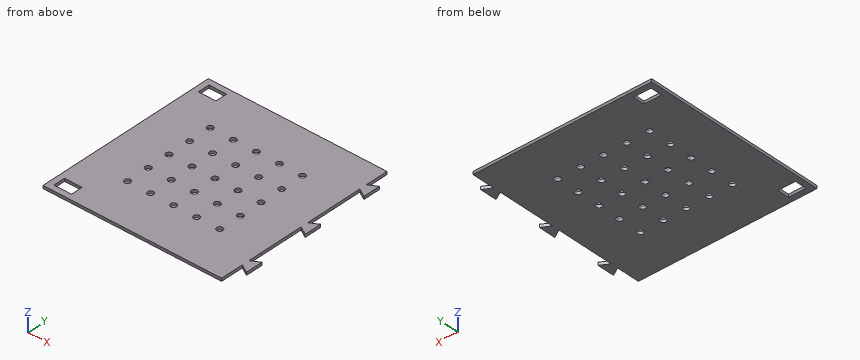
from build123d import *

# Parameters (mm, degrees)
SKETCH_W        = 155
SKETCH_H        = 160
PAD_DEPTH       = 2.5
SKETCH001_W     = 15.25
SKETCH001_H     = 10.25
POCKET_DEPTH    = 2.5
SKETCH002_R     = 2.625
POCKET001_DEPTH = 2.5
PAD001_DEPTH    = 2.5


with BuildPart() as part:
    # Sketch → Pad (new body)
    with BuildSketch(Plane.XY):
        with Locations((0.10674, -30.909095)):
            Rectangle(SKETCH_W, SKETCH_H)
    extrude(amount=PAD_DEPTH)

    # Sketch001 (on Face6 of Pad) → Pocket (cut)
    with BuildSketch(Plane.XY.offset(2.5)):
        with Locations((-64.76826, 38.965905)):
            Rectangle(SKETCH001_W, SKETCH001_H)
        with Locations((-64.76826, -100.784095)):
            Rectangle(SKETCH001_W, SKETCH001_H)
    extrude(amount=-POCKET_DEPTH, mode=Mode.SUBTRACT)

    # Sketch002 (on Face5 of Pocket) → Pocket001 (cut)
    with BuildSketch(Plane.XY.offset(2.5)):
        with Locations((-19.89326, -30.909095)):
            Circle(SKETCH002_R)
        with Locations((-39.89326, -30.909095)):
            Circle(SKETCH002_R)
        with Locations((0.10674, -30.909095)):
            Circle(SKETCH002_R)
        with Locations((20.10674, -30.909095)):
            Circle(SKETCH002_R)
        with Locations((40.10674, -30.909095)):
            Circle(SKETCH002_R)
        with Locations((-39.89326, -10.909095)):
            Circle(SKETCH002_R)
        with Locations((-19.89326, -10.909095)):
            Circle(SKETCH002_R)
        with Locations((0.10674, -10.909095)):
            Circle(SKETCH002_R)
        with Locations((20.10674, -10.909095)):
            Circle(SKETCH002_R)
        with Locations((40.10674, -10.909095)):
            Circle(SKETCH002_R)
        with Locations((-39.89326, -50.909095)):
            Circle(SKETCH002_R)
        with Locations((-19.89326, -50.909095)):
            Circle(SKETCH002_R)
        with Locations((0.10674, -50.909095)):
            Circle(SKETCH002_R)
        with Locations((20.10674, -50.909095)):
            Circle(SKETCH002_R)
        with Locations((40.10674, -50.909095)):
            Circle(SKETCH002_R)
        with Locations((-39.89326, -70.909095)):
            Circle(SKETCH002_R)
        with Locations((-19.89326, -70.909095)):
            Circle(SKETCH002_R)
        with Locations((0.10674, -70.909095)):
            Circle(SKETCH002_R)
        with Locations((20.10674, -70.909095)):
            Circle(SKETCH002_R)
        with Locations((40.10674, -70.909095)):
            Circle(SKETCH002_R)
        with Locations((-39.89326, 9.090905)):
            Circle(SKETCH002_R)
        with Locations((-19.89326, 9.090905)):
            Circle(SKETCH002_R)
        with Locations((0.10674, 9.090905)):
            Circle(SKETCH002_R)
        with Locations((20.10674, 9.090905)):
            Circle(SKETCH002_R)
        with Locations((40.10674, 9.090905)):
            Circle(SKETCH002_R)
    extrude(amount=-POCKET001_DEPTH, mode=Mode.SUBTRACT)

    # Sketch003 (on Face5 of Pocket001) → Pad001 (join)
    with BuildSketch(Plane.XY.offset(2.5)):
        Polygon((77.60674, -84.569349), (85.10674, -80.239222), (85.10674, -95.239222), (77.60674, -90.909095), align=None)
        Polygon((77.60674, -34.078841), (85.10674, -38.408968), (85.10674, -23.408968), (77.60674, -27.739095), align=None)
        Polygon((77.60674, 29.090905), (85.10674, 33.421032), (85.10674, 18.421032), (77.60674, 22.751159), align=None)
    extrude(amount=-PAD001_DEPTH)


solid = part.part
The model under review builds one solid part; all positions refer to its coordinate system, in mm. Round coordinates to 2 decimals unless told otherwise and drop trailing zeros. Write each loop counter-clockwise with the first axis right and the second up, starting at its lowest first coordinate (ties: lowest second). Pieces come first, ordered by that corner, then holes. Notation, with made-up numbers: M 59.5,80 L 76.5,80 A24 cw 76.5,99 Z; hole C 30,86.5 d4. An arc over 180 degrees is marked long. Use a Markdown table: item, result. Add a question column.
Q1. To check wall thickness, follow line 1 (Y direction, x = -61, z = 0.3); line 2 (X direction, y = 8.5, z = 1.8); line 3 (X direction, y = 38, z = 1.9). State the ranges of each line that lie inside material, in increasing order.
Q2. We need section A-A, the plane y = -101. State the section outline as (x, z) points.
Q3. Insertion check: pin 1 (4 mm diameter, centred on x = -19.89, y = 9.09, fed in from -Z); pin 2 (1.2 mm diameter, centred on y = -103, z = 1.5, fed in from +X). Each pin has a flat end and moves straight along its axis. Give the tip position at first contact, or say it passes through.
Q4. We need section D-D, the plane z = 1.2. Count the separate pieces of the cut face and the enclosed holes in it, plus the area to 3 significant figures.
Q5. We need section C-C, the plane x = 0. State the section outline as (y, z) points, plus the area to 3 significant figures.
Q6. We need section B-B, the plane x = -62. State the section outline as (y, z) points.
Findings below:
| question | item | result |
|---|---|---|
| 1 | line 1 | y = -110.91 to -105.91, -95.66 to 33.84, 44.09 to 49.09 |
| 1 | line 2 | x = -77.39 to -42.45, -37.34 to -22.45, -17.34 to -2.45, 2.66 to 17.55, 22.66 to 37.55, 42.66 to 77.61 |
| 1 | line 3 | x = -77.39 to -72.39, -57.14 to 77.61 |
| 2 | outline | M -77.39,0 L -72.39,0 L -72.39,2.5 L -77.39,2.5 Z; M -57.14,0 L 77.61,0 L 77.61,2.5 L -57.14,2.5 Z |
| 3 | pin 1 | passes through |
| 3 | pin 2 | stops at x = 77.61 |
| 4 | separate pieces | 1 |
| 4 | enclosed holes | 27 |
| 4 | area | 24,200 mm² |
| 5 | outline | M -110.91,0 L -73.53,0 L -73.53,2.5 L -110.91,2.5 Z; M -68.29,0 L -53.53,0 L -53.53,2.5 L -68.29,2.5 Z; M -48.29,0 L -33.53,0 L -33.53,2.5 L -48.29,2.5 Z; M -28.29,0 L -13.53,0 L -13.53,2.5 L -28.29,2.5 Z; M -8.29,0 L 6.47,0 L 6.47,2.5 L -8.29,2.5 Z; M 11.71,0 L 49.09,0 L 49.09,2.5 L 11.71,2.5 Z |
| 5 | area | 334 mm² |
| 6 | outline | M -110.91,0 L -105.91,0 L -105.91,2.5 L -110.91,2.5 Z; M -95.66,0 L 33.84,0 L 33.84,2.5 L -95.66,2.5 Z; M 44.09,0 L 49.09,0 L 49.09,2.5 L 44.09,2.5 Z |
